Input: part model. Units: mm. Frame: model coordinates. A direction names the side the tool comes from. Coordinates: 2 decimals unless noted, no trailing zeros. Write each loop counter-clockwise with the first axis right and the second up, starting at its lowest first coordinate (ties: lowest second). Pieces come first, ordered by that corner, then holes. Notation, with made-up numbers: (-3.5, -14.5) -> (49.5, -14.5) arc R23 ccw to (49.5, 24.5) -> close; hole circle Ø10 at (64.5, -27.5). An arc over 180 degrees is marked (long way). One line per question, with ' | ' between items. Start each with the question number.
```python
from build123d import *

# Parameters (mm, degrees)
BOSS_EXTRUDE1_DEPTH = 8.5
SKETCH2_W           = 16.5
SKETCH2_H           = 13
CUT_EXTRUDE1_DEPTH  = 16.5
CUT_EXTRUDE2_DEPTH  = 3.5
CUT_EXTRUDE3_DEPTH  = 3.5


with BuildPart() as part:
    # Sketch1 → Boss-Extrude1 (new body, symmetric)
    with BuildSketch(Plane(origin=(0, 0, 0), x_dir=(1, 0, 0), z_dir=(0, 1, 0))):
        with BuildLine():
            Line((0, 20), (0, 0))
            Line((0, 0), (-20, 0))
            Line((-20, 0), (-20, 3.5))
            ThreePointArc((-20, 3.5), (-13.435028843, 13.435028843), (-3.5, 20))
            Line((-3.5, 20), (0, 20))
        make_face()
    extrude(amount=BOSS_EXTRUDE1_DEPTH, both=True)

    # Sketch2 → Cut-Extrude1 (cut)
    with BuildSketch(Plane.ZY.offset(20)):
        with Locations((-11.75, 0)):
            Rectangle(SKETCH2_W, SKETCH2_H)
    extrude(amount=-CUT_EXTRUDE1_DEPTH, mode=Mode.SUBTRACT)

    # Sketch4 → Cut-Extrude2 (cut)
    with BuildSketch(Plane.XY):
        with BuildLine():
            Line((-7.25, 2.75), (-12.75, 2.75))
            ThreePointArc((-12.75, 2.75), (-15.5, 0), (-12.75, -2.75))
            Line((-12.75, -2.75), (-7.25, -2.75))
            ThreePointArc((-7.25, -2.75), (-4.5, 0), (-7.25, 2.75))
        make_face()
    extrude(amount=-CUT_EXTRUDE2_DEPTH, mode=Mode.SUBTRACT)

    # Sketch5 → Cut-Extrude3 (cut)
    with BuildSketch(Plane(origin=(0, 0, 0), x_dir=(0, 0, -1), z_dir=(1, 0, 0))):
        with BuildLine():
            Line((7.25, 2.75), (12.75, 2.75))
            ThreePointArc((12.75, 2.75), (15.5, 0), (12.75, -2.75))
            Line((12.75, -2.75), (7.25, -2.75))
            ThreePointArc((7.25, -2.75), (4.5, 0), (7.25, 2.75))
        make_face()
    extrude(amount=-CUT_EXTRUDE3_DEPTH, mode=Mode.SUBTRACT)


solid = part.part
```
1) Section A-A, the plane x = -3. Return loops of the section in (y, z).
2) Section B-B, the plane y = 0. Return loops of the section in (x, z), then the cut area to 4 significant figures.
3) Pull-direction query (Z, two-part tool) for faces 1 (the face through (-2, 2.75, -10)), 2 (the face through (-10, -6.5, -10)), 3 (the face through (-13.55, 7.51, -13.32)), 4 (the face through (-1.7, 0.1, -15.5)); classes: released by +Z, released by -Z, zero draft, split by the parting line, or undercut.
4) Section C-C, the plane z = -1.5. Return loops of the section in (x, y), then the cut area to 3 significant figures.
5) Access query for faces 5 (the face through (-8, -8.5, -8)), 6 (the face through (-2, -2.75, -10)), 7 (the face through (-4.5, -0.1, -1.7)), 8 (the face through (-3.5, 3, -12)). Directions: +Z, -Z, +X, -X, +Y, -Y. A direction counts if a zero-diameter tool reaches every point of the face in a straight line with its end or side. Return the directions, or none.
6) First-contact query: P1, Ø1.5, axis at y = 1, z = -14, coming from the +X side. Flat tip, straight axial feed; report the tip coordinate or a pass-through.
7) Ray query, line 1 (Y direction, x = -11, z = -6.5); line 2 (Y direction, x = -7.25, z = -1.5); line 3 (Z direction, x = -9.25, y = 6). Return the intervals inside material, ascending.
8) Section D-D, the plane z = -6. Return loops of the section in (x, y), then the cut area to 3 significant figures.
Answer block:
1) outline: (-8.5, -20) -> (8.5, -20) -> (8.5, 0) -> (-8.5, 0) -> close; hole (-2.75, -12.75) arc R2.75 ccw to (2.75, -12.75) -> (2.75, -7.25) arc R2.75 ccw to (-2.75, -7.25) -> close
2) outline: (-20, -3.5) -> (-15.5, -3.5) -> (-15.5, 0) -> (-20, 0) -> close; (-4.5, -3.5) -> (-3.5, -3.5) -> (-3.5, -4.5) -> (0, -4.5) -> (0, 0) -> (-4.5, 0) -> close; (-3.5, -20) -> (0, -20) -> (0, -15.5) -> (-3.5, -15.5) -> close | area: 50.75 mm2
3) face 1: undercut | face 2: zero draft | face 3: released by -Z | face 4: undercut
4) outline: (-20, -8.5) -> (0, -8.5) -> (0, 8.5) -> (-20, 8.5) -> close; hole (-12.75, -2.75) -> (-7.25, -2.75) arc R2.75 ccw to (-7.25, 2.75) -> (-12.75, 2.75) arc R2.75 ccw to start | area: 286 mm2
5) face 5: +Z, -Z, +X, -X, -Y | face 6: +X, -X | face 7: +Z, -Z | face 8: -Z, -X
6) P1: passes through
7) line 1: y = -8.5 to -6.5, 6.5 to 8.5 | line 2: y = -8.5 to -2.75, 2.75 to 8.5 | line 3: z = -3.5 to 0
8) outline: (-18.86, -8.5) -> (0, -8.5) -> (0, -2.45) -> (-3.5, -2.45) -> (-3.5, -6.5) -> (-18.86, -6.5) -> close; (-18.86, 6.5) -> (-3.5, 6.5) -> (-3.5, 2.45) -> (0, 2.45) -> (0, 8.5) -> (-18.86, 8.5) -> close | area: 104 mm2
